Design review of the part built by this model. Coordinates are the model's own, in mm. A direction names the side the tool comes from. Coordinates: 2 decimals unless noted, no trailing zeros. Write each loop counter-clockwise with the first axis right and the second up, starting at its lowest first coordinate (ties: lowest second). Pieces come first, ordered by that corner, then holes. Notation, with made-up numbers: (73, 75.5) - (90, 75.5) arc R29 ccw to (90, 106.5) - close; hole circle Ø3 at (38.5, 66.5). An arc over 180 degrees is marked (long way). One line per item, written item: value.
from build123d import *

# Parameters (mm, degrees)
BOSS_EXTRUDE1_DEPTH = 6
SKETCH2_R           = 57.07
BOSS_EXTRUDE2_DEPTH = 39
CUT_EXTRUDE1_START  = -35.8
SKETCH3_R           = 57.07
SKETCH3_R_2         = 55.591
CUT_EXTRUDE1_DEPTH  = 35.8


with BuildPart() as part:
    # Sketch1 → Boss-Extrude1 (new body)
    with BuildSketch(Plane(origin=(0, 0, 0), x_dir=(0, 0, -1), z_dir=(1, 0, 0))):
        Polygon((33.053302911, 57.25), (-33.053302911, 57.25), (-66.106605822, 0), (-33.053302911, -57.25), (33.053302911, -57.25), (66.106605822, 0), align=None)
    extrude(amount=BOSS_EXTRUDE1_DEPTH)

    # Sketch2 → Boss-Extrude2 (add)
    with BuildSketch(Plane(origin=(6, 0, 0), x_dir=(0, 0, -1), z_dir=(1, 0, 0))):
        Circle(SKETCH2_R)
    extrude(amount=BOSS_EXTRUDE2_DEPTH)

    # Sketch3 → Cut-Extrude1 (cut)
    with BuildSketch(Plane(origin=(45, 0, 0), x_dir=(0, 0, -1), z_dir=(1, 0, 0)).offset(CUT_EXTRUDE1_START)):
        Circle(SKETCH3_R)
        Circle(SKETCH3_R_2, mode=Mode.SUBTRACT)
    extrude(amount=CUT_EXTRUDE1_DEPTH, mode=Mode.SUBTRACT)


solid = part.part
1. Consider section C-C, the plane x = 36.5. Write out the cut boundary in (y, z).
Answer block:
outline: circle Ø111.18 at (0, 0)
2. For faces 1 (the face through (2.958, -28.224, 49.811)), 2 (the face through (26.85, -54.27, 12.05)), list the 3-axis set-ups (+Z, -Z, +X, -X, +Y, -Y) from which the entire face can be reached by the end or side of a thin tool; tool diameter is ignored.
Answer block:
face 1: +Z, +X, -X, -Y
face 2: +X
3. Consider section B-B, the plane y = -3.5. Write out the cut boundary in (x, z), then the cut area to 3 significant figures.
Answer block:
outline: (0, -64.09) - (6, -64.09) - (6, -56.96) - (9.2, -56.96) - (9.2, -55.48) - (45, -55.48) - (45, 55.48) - (9.2, 55.48) - (9.2, 56.96) - (6, 56.96) - (6, 64.09) - (0, 64.09) - close
area: 5,110 mm^2
4. Mouldability with a two-part tool opening along Y and no side actions: class faces 3 (the face through (7.578, 17.142, -54.435)), 4 (the face through (2.958, 29.026, 49.349)), 5 (the face through (9.2, -55, -12)) as released by +Y, released by -Y, zero draft, split by the parting line, or undercut.
Answer block:
face 3: split by the parting line
face 4: released by +Y
face 5: zero draft
5. Wall thickness on line 1 along Z through (x, y) = (20.5, 21); line 2 along Z through (x, y) = (16.5, 16.5); line 3 along Y through (x, z) = (8.5, -11): over which ranges is each line inside the solid? List them lowest first.
Answer block:
line 1: z = -51.47 to 51.47
line 2: z = -53.09 to 53.09
line 3: y = -56 to 56
6. Insertion check: pin 1 Ø1.5 at (x, y) = (18.5, -44) entering from -Z; pin 2 Ø1 at (x, z) = (26, 5) entering from -Y; pin 3 Ø4 at (x, z) = (9.5, 23) entering from +Y. Each pin has a flat end and moves straight along its axis. Give the tip position at first contact, or say it passes through.
Answer block:
pin 1: stops at z = -34.93
pin 2: stops at y = -55.41
pin 3: stops at y = 53.06
7. Consider section A-A, the plane z = 14.5. Write out the cut boundary in (x, y).
Answer block:
outline: (0, -57.25) - (6, -57.25) - (6, -55.2) - (9.2, -55.2) - (9.2, -53.67) - (45, -53.67) - (45, 53.67) - (9.2, 53.67) - (9.2, 55.2) - (6, 55.2) - (6, 57.25) - (0, 57.25) - close
